The model under review builds one solid part; all positions refer to its coordinate system, in mm. Round coordinates to 2 decimals unless told otherwise and drop trailing zeros. Order: outer loops, then holes, each group sorted by start corner. A loop starts at its lowest first (then second) coordinate and runs counter-clockwise, first axis right, second up. Notation, with made-up numbers: (3, 29) -> (31, 29) arc R37 ccw to (31, 68) -> close; hole circle Ø8 at (48, 62.25). An arc over 180 degrees is marked (long way). Use a Markdown table: item, result. Add a question column.
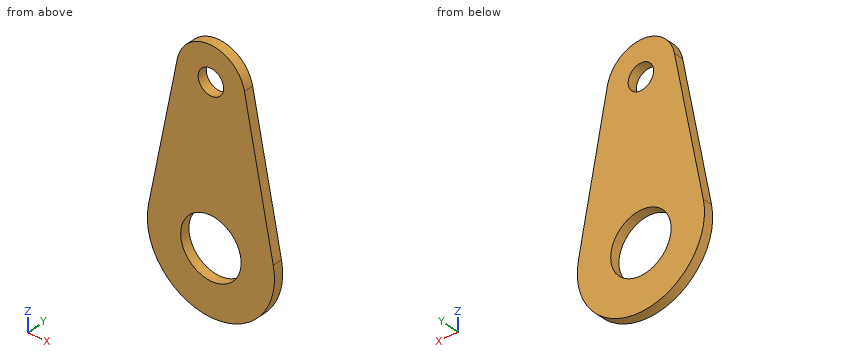
```python
from build123d import *

# Parameters (mm, degrees)
SKETCH1_R               = 3.999999916
BOSS_EXTRUDE1_DEPTH     = 3
CUT_EXTRUDE3_DEPTH      = 14052.939444196
CUT_EXTRUDE3_DEPTH_BACK = 14052.939444196
SKETCH3_R               = 9.5


with BuildPart() as part:
    # Sketch1 → Boss-Extrude1 (new body)
    with BuildSketch(Plane(origin=(0, 0, 0), x_dir=(1, 0, 0), z_dir=(0, 1, 0))):
        with BuildLine():
            Line((-13667.630300179, 3154.015259161), (-13676.700320557, 3200.215044723))
            ThreePointArc((-13676.700320557, 3200.215044723), (-13657.074947978, 3224.067930782), (-13637.449575399, 3200.215044723))
            Line((-13637.449575399, 3200.215044723), (-13646.519595777, 3154.015259161))
            ThreePointArc((-13646.519595777, 3154.015259161), (-13657.074947978, 3145.314842225), (-13667.630300179, 3154.015259161))
        make_face()
        with Locations(Location((-13657.074947978, 3156.067931204, 0), (0, 0, 269.999999999))):
            Circle(SKETCH1_R, mode=Mode.SUBTRACT)
        Polygon((-13663.074951578, 3198.067969394), (-13651.074950322, 3198.067909928), (-13651.074919654, 3210.067922748), (-13663.074916837, 3210.067922748), align=None, mode=Mode.SUBTRACT)
    extrude(amount=BOSS_EXTRUDE1_DEPTH)

    # Sketch3 → Cut-Extrude3 (cut, two sides: drawn at the far end of the back side and taken through both)
    with BuildSketch(Plane.XZ.offset(-CUT_EXTRUDE3_DEPTH_BACK)):
        with Locations(Location((-13657.07493358, -3204.067916338, 0), (0, 0, 270))):
            Circle(SKETCH3_R)
    extrude(amount=CUT_EXTRUDE3_DEPTH + CUT_EXTRUDE3_DEPTH_BACK, mode=Mode.SUBTRACT)


solid = part.part
```
Q1. For pin 1 (1.5 mm diameter, centred on x = -13659.5, y = 1.5, fed in from -Z); pin 2 (1 mm diameter, centred on x = -13667.5, y = 2, fed in from -Z); pin 3 (1 mm diameter, centred on x = -13656, y = 1.5, fed in from +Z), all flat-tipped, find the tip position at first contact; note any pin that passes through.
Q2. Add section A-A, the plane z = -3209. Give the boundary of the cut face in (x, y), then the cut area to 3 significant figures.
Q3. To check wall thickness, follow line 1 along Z through (x, y) = (-13658.5, 2.5); line 2 along Z through (x, y) = (-13659, 1.95) (3 decimals); line 3 along Z through (x, y) = (-13648.5, 0.9). State the ranges of each line that lie inside material, in increasing order.
Q4. Add section B-B, the plane x = -13655. Give the boundary of the cut face in (y, z), then the cut area to 3 significant figures.
Q5. Add section C-C, the plane x = -13665.5. Give the boundary of the cut face in (y, z), then the cut area to 3 significant figures.
Q6. Add section D-D, the plane y = 1.7. Give the boundary of the cut face in (x, z), then the cut area to 3 significant figures.
Return value:
| question | item | result |
|---|---|---|
| 1 | pin 1 | z = -3224 |
| 1 | pin 2 | z = -3221.43 |
| 1 | pin 3 | z = -3145.33 |
| 2 | outline | (-13676.46, 0) -> (-13665.19, 0) -> (-13665.19, 3) -> (-13676.46, 3) -> close; (-13648.96, 0) -> (-13637.69, 0) -> (-13637.69, 3) -> (-13648.96, 3) -> close |
| 2 | area | 67.6 mm² |
| 3 | line 1 | -3224.02 to -3213.46, -3194.68 to -3159.81, -3152.33 to -3145.41 |
| 3 | line 2 | -3223.975 to -3213.371, -3194.765 to -3159.574, -3152.562 to -3145.489 |
| 3 | line 3 | -3222.14 to -3208.16, -3199.98 to -3149.58 |
| 4 | outline | (0, -3223.96) -> (3, -3223.96) -> (3, -3213.34) -> (0, -3213.34) -> close; (0, -3194.8) -> (3, -3194.8) -> (3, -3159.49) -> (0, -3159.49) -> close; (0, -3152.65) -> (3, -3152.65) -> (3, -3145.52) -> (0, -3145.52) -> close |
| 4 | area | 159 mm² |
| 5 | outline | (0, -3222.21) -> (3, -3222.21) -> (3, -3208.46) -> (0, -3208.46) -> close; (0, -3199.68) -> (3, -3199.68) -> (3, -3149.39) -> (0, -3149.39) -> close |
| 5 | area | 192 mm² |
| 6 | outline | (-13676.7, -3200.22) arc R20 ccw (long way) to (-13637.45, -3200.22) -> (-13646.52, -3154.02) arc R10.75 ccw to (-13667.63, -3154.02) -> close; hole circle Ø19 at (-13657.07, -3204.07); hole circle Ø8 at (-13657.07, -3156.07) |
| 6 | area | 1,980 mm² |
